Model file for the job. Use its own axes, mm. Face numbers are marked on the shaded views. A direction names the side the tool comes from. Coordinates: 2 decimals unless noted, no trailing zeros. Write each loop counter-clockwise with the first axis right and the second up, starting at its lowest first coordinate (ties: lowest second). Pieces come first, ordered by that corner, then holes. Notation, with made-up numbers: (17, -30) - (26, -30) arc R34 cw to (26, 3) - close; hole circle Ø1 at (86, 41). An arc over 180 degrees is marked (long way). Put each result on its own line as item: value. Start each with the question number.
1. Pull direction Y, two halves, no side cores. Call the marked faces 6, 7, 8 and 9: released by +Y, released by -Y, zero draft, split by the parting line, or undercut.
2. Which spindle directions (+Z, -Z, +X, -X, +Y, -Y) get a long thin tool onto all of the face, cutting with end or side? Do the marked faces 1, 2, 3, 4 and 5. Say none if no direction does.
3. Drop flat-ended pins along their axis: P1, Ø2, axis at y = 23.5, z = 5.5, coming from the -X side; P2, Ø14.5, axis at x = 13.24, y = 4.12, coming from the +Z side; P3, Ø1.9, axis at x = -26.5, z = 4.5, coming from the -Y side; P4, Ø2, axis at y = 17, z = 3.5, coming from the +X side. Give the stop position or say it passes through.
4. Drill centre lines: L1, parallel to X at y = 38, z = 4; L2, parallel to Y at x = 43, z = 4.5; L3, parallel to X at y = 4.5, z = 4.5. Where is each one in solid material? Low to high. Write a range as from..to.
5. Saw through at A-A, the plane y = 20.5. Write the cut outline in (x, z), plus the area to 3 significant figures.
6. Saw through at B-B, the plane x = 5.5. Write the cut outline in (y, z).
7. Saw through at C-C, the plane z = 2.75. Give the number of separate pieces and of enclosed holes in the cut face, plus the area to 3 significant figures.
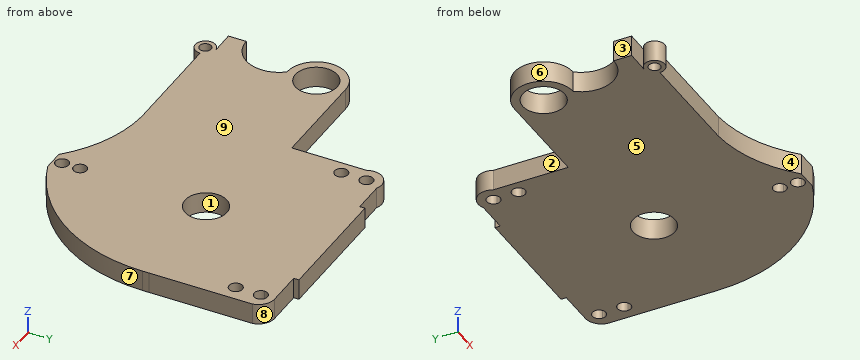
```python
from build123d import *

# Parameters (mm, degrees)
F0_R     = 1.778
F0_R_2   = 6.35
F0_W     = 38.1
F0_H     = 1.5911871894
F1_DEPTH = 6.35


with BuildPart() as f1:
    # F0 (on Top) → F1 (new body)
    with BuildSketch(Plane.XY):
        with BuildLine():
            Line((16.4140281489, -30.8064179522), (16.4140281489, -30.6620997704))
            ThreePointArc((16.4140281489, -30.6620997704), (38.6980048273, -19.7929887048), (48.1532220223, 3.1266984605))
            Line((48.1532220223, 3.1266984605), (48.1532220223, 5.1104656351))
            ThreePointArc((48.1532220223, 5.1104656351), (44.4486160884, 19.800484772), (34.8719360944, 31.5396486119))
            Line((34.8719360944, 31.5396486119), (32.2923098035, 36.5656356997))
            Line((32.2923098035, 36.5656356997), (32.2923098035, 40.7379940159))
            Line((32.2923098035, 40.7379940159), (-5.8076901965, 40.7379940159))
            Line((-5.8076901965, 40.7379940159), (-5.8076901965, 36.5656356997))
            Line((-5.8076901965, 36.5656356997), (-8.3873164875, 31.5396486119))
            ThreePointArc((-8.3873164875, 31.5396486119), (-18.0627806357, 19.7145570203), (-21.7750586109, 4.893410308))
            ThreePointArc((-21.7750586109, 4.893410308), (-21.4769400323, -0.6314389882), (-20.311434257, -6.0401755062))
            ThreePointArc((-20.311434257, -6.0401755062), (-16.1913746397, -14.967065801), (-9.7499520252, -22.3948741107))
            Line((-9.7499520252, -22.3948741107), (-52.8449263588, -22.3948741107))
            Line((-52.8449263588, -22.3948741107), (-60.4649263588, -22.3948741107))
            Line((-60.4649263588, -22.3948741107), (-60.4649263588, -27.8276202867))
            Line((-60.4649263588, -27.8276202867), (-52.9002836607, -27.758920689))
            ThreePointArc((-52.9002836607, -27.758920689), (-54.980526385, -32.9811631161), (-49.7969263588, -30.8064179522))
            Line((-49.7969263588, -30.8064179522), (-19.8648082777, -30.8064179522))
            ThreePointArc((-19.8648082777, -30.8064179522), (-17.9420934961, -30.7601008655), (-16.0193787145, -30.8064179522))
            Line((-16.0193787145, -30.8064179522), (10.0673098035, -30.8064179522))
            Line((10.0673098035, -30.8064179522), (13.2406689762, -30.8064179522))
            Line((13.2406689762, -30.8064179522), (16.4140281489, -30.8064179522))
        make_face()
        with Locations((-52.8449263588, -30.8064179522)):
            Circle(F0_R, mode=Mode.SUBTRACT)
        with Locations((13.2423098035, 4.1185820478)):
            Circle(F0_R_2, mode=Mode.SUBTRACT)
        with BuildLine():
            ThreePointArc((48.1532220223, 3.1266984605), (38.6980048273, -19.7929887048), (16.4140281489, -30.6620997704))
            Line((16.4140281489, -30.6620997704), (16.4140281489, -30.8064179522))
            Line((16.4140281489, -30.8064179522), (16.4140281489, -42.2313285658))
            ThreePointArc((16.4140281489, -42.2313285658), (39.4304466926, -24.5532899944), (48.1532220223, 3.1266984605))
        make_face()
        with BuildLine():
            Line((48.1532220223, 5.1104656351), (48.1532220223, 3.1266984605))
            ThreePointArc((48.1532220223, 3.1266984605), (48.1673098035, 4.1185820478), (48.1532220223, 5.1104656351))
        make_face()
        with BuildLine():
            Line((16.4140281489, -42.2313285658), (16.4140281489, -30.8064179522))
            Line((16.4140281489, -30.8064179522), (13.2406689762, -30.8064179522))
            Line((13.2406689762, -30.8064179522), (13.2406689762, -32.0282139509))
            ThreePointArc((13.2406689762, -32.0282139509), (14.6746436477, -32.6221857079), (15.2686154047, -34.0561603794))
            ThreePointArc((15.2686154047, -34.0561603794), (14.6746436477, -35.4901350508), (13.2406689762, -36.0841068079))
            Line((13.2406689762, -36.0841068079), (13.2406689762, -37.5133532824))
            ThreePointArc((13.2406689762, -37.5133532824), (14.6775099555, -38.108512303), (15.2726689762, -39.5453532824))
            ThreePointArc((15.2726689762, -39.5453532824), (14.6775099555, -40.9821942618), (13.2406689762, -41.5773532824))
            Line((13.2406689762, -41.5773532824), (13.2406689762, -42.2313285658))
            Line((13.2406689762, -42.2313285658), (16.4140281489, -42.2313285658))
        make_face()
        with BuildLine():
            ThreePointArc((34.8719360944, 31.5396486119), (44.4486160884, 19.800484772), (48.1532220223, 5.1104656351))
            Line((48.1532220223, 5.1104656351), (48.1532220223, 36.5656356997))
            ThreePointArc((48.1532220223, 36.5656356997), (46.5024271992, 39.5513463721), (43.3037619874, 40.7379940159))
            Line((43.3037619874, 40.7379940159), (32.2923098035, 40.7379940159))
            Line((32.2923098035, 40.7379940159), (32.2923098035, 36.5656356997))
            Line((32.2923098035, 36.5656356997), (34.8719360944, 31.5396486119))
        make_face()
        with BuildLine():
            ThreePointArc((45.3357619874, 28.9456356997), (41.866921008, 27.5087947203), (43.3037619874, 30.9776356997))
            ThreePointArc((43.3037619874, 30.9776356997), (44.7406029667, 30.3824766791), (45.3357619874, 28.9456356997))
        make_face(mode=Mode.SUBTRACT)
        with BuildLine():
            ThreePointArc((43.3037619874, 34.5336356997), (41.866921008, 35.1287947203), (41.2717619874, 36.5656356997))
            ThreePointArc((41.2717619874, 36.5656356997), (43.3037619874, 38.5976356997), (45.3357619874, 36.5656356997))
            ThreePointArc((45.3357619874, 36.5656356997), (44.7406029667, 35.1287947203), (43.3037619874, 34.5336356997))
        make_face(mode=Mode.SUBTRACT)
        with BuildLine():
            Line((13.2406689762, -32.0282139509), (13.2406689762, -30.8064179522))
            Line((13.2406689762, -30.8064179522), (10.0673098035, -30.8064179522))
            Line((10.0673098035, -30.8064179522), (10.0673098035, -42.2313285658))
            Line((10.0673098035, -42.2313285658), (13.2406689762, -42.2313285658))
            Line((13.2406689762, -42.2313285658), (13.2406689762, -41.5773532824))
            ThreePointArc((13.2406689762, -41.5773532824), (11.2086689762, -39.5453532824), (13.2406689762, -37.5133532824))
            Line((13.2406689762, -37.5133532824), (13.2406689762, -36.0841068079))
            ThreePointArc((13.2406689762, -36.0841068079), (11.2127225477, -34.0561603794), (13.2406689762, -32.0282139509))
        make_face()
        with BuildLine():
            Line((10.0673098035, -42.2313285658), (10.0673098035, -30.8064179522))
            Line((10.0673098035, -30.8064179522), (-16.0193787145, -30.8064179522))
            ThreePointArc((-16.0193787145, -30.8064179522), (-1.9228841261, -34.1141975872), (10.0673098035, -42.2313285658))
        make_face()
        with BuildLine():
            Line((-19.8648082777, -30.8064179522), (-16.0193787145, -30.8064179522))
            ThreePointArc((-16.0193787145, -30.8064179522), (-17.9420934961, -30.7601008655), (-19.8648082777, -30.8064179522))
        make_face()
        with Locations((13.2423098035, 41.5335876106)):
            Rectangle(F0_W, F0_H)
        with BuildLine():
            Line((-5.8076901965, 36.5656356997), (-5.8076901965, 40.7379940159))
            Line((-5.8076901965, 40.7379940159), (-15.5782827911, 40.7379940159))
            Line((-15.5782827911, 40.7379940159), (-19.681555644, 40.7379940159))
            ThreePointArc((-19.681555644, 40.7379940159), (-22.040670707, 38.0363692731), (-21.7750586109, 34.4595480103))
            Line((-21.7750586109, 34.4595480103), (-21.7750586109, 11.7398244938))
            Line((-21.7750586109, 11.7398244938), (-21.7750586109, 4.893410308))
            ThreePointArc((-21.7750586109, 4.893410308), (-18.0627806357, 19.7145570203), (-8.3873164875, 31.5396486119))
            Line((-8.3873164875, 31.5396486119), (-5.8076901965, 36.5656356997))
        make_face()
        with BuildLine():
            ThreePointArc((-15.5979192176, 28.9456356997), (-19.0667601969, 27.5087947203), (-17.6299192176, 30.9776356997))
            ThreePointArc((-17.6299192176, 30.9776356997), (-16.1930782382, 30.3824766791), (-15.5979192176, 28.9456356997))
        make_face(mode=Mode.SUBTRACT)
        with BuildLine():
            ThreePointArc((-17.6299192176, 34.5336356997), (-19.0667601969, 38.0024766791), (-15.5979192176, 36.5656356997))
            ThreePointArc((-15.5979192176, 36.5656356997), (-16.1930782382, 35.1287947203), (-17.6299192176, 34.5336356997))
        make_face(mode=Mode.SUBTRACT)
        with BuildLine():
            Line((-19.681555644, 40.7379940159), (-15.5782827911, 40.7379940159))
            ThreePointArc((-15.5782827911, 40.7379940159), (-17.6299192176, 41.2151287844), (-19.681555644, 40.7379940159))
        make_face()
        with BuildLine():
            ThreePointArc((-20.311434257, -6.0401755062), (-21.4769400323, -0.6314389882), (-21.7750586109, 4.893410308))
            Line((-21.7750586109, 4.893410308), (-21.7750586109, 11.7398244938))
            Line((-21.7750586109, 11.7398244938), (-52.8400652111, 11.7398244938))
            ThreePointArc((-52.8400652111, 11.7398244938), (-61.7300652111, 2.8498244938), (-52.8400652111, -6.0401755062))
            Line((-52.8400652111, -6.0401755062), (-20.311434257, -6.0401755062))
        make_face()
        with Locations((-52.8400652111, 2.8498244938)):
            Circle(F0_R_2, mode=Mode.SUBTRACT)
        with BuildLine():
            ThreePointArc((-52.8400652111, -6.0401755062), (-51.4425282025, -16.6465074734), (-60.4649263588, -22.3948741107))
            Line((-60.4649263588, -22.3948741107), (-52.8449263588, -22.3948741107))
            Line((-52.8449263588, -22.3948741107), (-9.7499520252, -22.3948741107))
            ThreePointArc((-9.7499520252, -22.3948741107), (-16.1913746397, -14.967065801), (-20.311434257, -6.0401755062))
            Line((-20.311434257, -6.0401755062), (-52.8400652111, -6.0401755062))
        make_face()
    extrude(amount=F1_DEPTH)


solid = f1.part
```
Final values:
1. face 6: undercut
1. face 7: released by -Y
1. face 8: released by +Y
1. face 9: zero draft
2. face 1: +Z, -Z
2. face 2: +Z, -Z, -X
2. face 3: +Z, -Z, -X, -Y
2. face 4: +Z, -Z, -Y
2. face 5: -Z, +X, -X, +Y, -Y
3. P1: stops at x = -21.78
3. P2: stops at z = 6.35
3. P3: stops at y = -30.81
3. P4: stops at x = 48.15
4. L1: x = -22.05..-19.07, -16.19..41.86, 44.74..47.7
4. L2: y = -18.58..26.94, 30.95..34.56, 38.57..40.74
4. L3: x = -61.58..-58.97, -46.71..6.9, 19.58..48.17
5. outline: (-21.78, 0) - (48.15, 0) - (48.15, 6.35) - (-21.78, 6.35) - close
5. area: 444 mm²
6. outline: (-38.37, 0) - (42.33, 0) - (42.33, 6.35) - (-38.37, 6.35) - close
7. separate pieces: 1
7. enclosed holes: 9
7. area: 6,360 mm²
